Design review of the part built by this model. Coordinates are the model's own, in mm. A direction names the side the tool comes from. Coordinates: 2 decimals unless noted, no trailing zeros. Loops run counter-clockwise (first coordinate to the right, second up) from the corner with the lowest first, then second, coordinate; pieces in that order, holes last. Notation, with made-up numbers: (81.5, 37) - (89.5, 37) arc R16 ccw to (89.5, 55) - close; hole circle Ø8 at (70, 7.5). An arc over 180 degrees is marked (long way). Use one line per item in the form item = value. Start each with the question number.
(1) Add section A-A (z = 14). Count the separate pieces of the cut face and the enclosed holes in it, plus the area to 3 significant figures.
(2) Tool access review of faces 4 (the face through (0.81, 19.37, 26.5)), 5 (the face through (60.85, 1, 14)), 6 (the face through (78.4, 12, 14)): name each direction out of +Z, -Z, +X, -X, +Y, -Y from which nothing blocks a thin tool from reaching the whole face with its end or side.
(3) Add section C-C (x = 39.5). State the section outline as (y, z) points.
(4) The part is to be moulded in two halves that separate along Y. For faces 1 (the face through (39, 1.6, 26)), 2 (the face through (79.189, 14.097, 14.631)), 3 (the face through (0.782, 0.741, 13.804)), say which applies: pulls with the +Y half, pulls with the -Y half, needs draft (parallel to the pull), parting line crosses it, or undercut.
(5) For L1, parallel to Z at x = 78.8, y = 8.1; L2, parallel to X at y = 5, z = 21; L3, parallel to X at y = 1.5, z = 9, list the stretches that pass through material, from the lowest coordinate up.
(6) Clearance check with flat-ended pins moving along their axes: pin 1 Ø4 at (x, z) = (70, 12.5) entering from +Y; pin 2 Ø1.3 at (y, z) = (1, 10) entering from +X; pin 3 Ø5.5 at (x, z) = (65, 18.9) entering from -Y; pin 4 Ø0.8 at (y, z) = (1, 19) entering from +X. State where each tip first meets the part, or that it passes through.
(7) Add section B-B (y = 3.5). State the section outline as (x, z) points, plus the area to 3 significant figures.
(8) Add section D-D (x = 65). State the section outline as (y, z) points, plus the area to 3 significant figures.
```python
from build123d import *

# Parameters (mm, degrees)
SKETCH1_W                      = 80
SKETCH1_H                      = 28
BOSS_EXTRUDE1_DEPTH            = 1.6
SKETCH2_R                      = 2.1
CUT_EXTRUDE1_DEPTH             = 85.77358079
LPATTERN1_COUNT                = 2
LPATTERN1_PITCH                = 50
LPATTERN1_COUNT_DIR2           = 2
LPATTERN1_PITCH_DIR2           = 9.8
SKETCH15_W                     = 41.7
SKETCH15_H                     = 21
CUT_EXTRUDE3_DEPTH             = 85.77358079
EDGE_FLANGE1_STRIP_W           = 8.4
EDGE_FLANGE1_STRIP_H           = 1.6
EDGE_FLANGE1_STRIP_CUT_DEPTH   = 28
EDGE_FLANGE1_STRIP_2_W         = 8.4
EDGE_FLANGE1_STRIP_2_H         = 1.6
EDGE_FLANGE1_STRIP_CUT_2_DEPTH = 28
EDGE_FLANGE1_DEPTH             = 28
EDGE_FLANGE1_BEND_DEPTH        = 28
FILLET1_R                      = 5
SKETCH14_R                     = 2.1
CUT_EXTRUDE2_DEPTH             = 88.273363634
LPATTERN2_COUNT                = 3
LPATTERN2_PITCH                = 8
LPATTERN2_COUNT_DIR2           = 2
LPATTERN2_PITCH_DIR2           = 8
CUT_EXTRUDE4_DEPTH             = 10


# Sheet-metal steps are written as plain solids
with BuildPart() as part:
    # Sketch1 → Boss-Extrude1 (new body)
    with BuildSketch(Plane(origin=(0, 0, 0), x_dir=(1, 0, 0), z_dir=(0, 1, 0))):
        with Locations((40, -14)):
            Rectangle(SKETCH1_W, SKETCH1_H)
    extrude(amount=BOSS_EXTRUDE1_DEPTH)

    # Sketch2 → Cut-Extrude1 (cut, through all)
    with BuildSketch(Plane(origin=(0, 1.6, 0), x_dir=(1, 0, 0), z_dir=(0, 1, 0))):
        with Locations(Location((15, -9.1, 0), (0, 0, 270))):
            Circle(SKETCH2_R)
    cut_extrude1 = extrude(amount=-CUT_EXTRUDE1_DEPTH, mode=Mode.SUBTRACT)

    # LPattern1: Cut-Extrude1 2 × 2
    with Locations(*[(i * LPATTERN1_PITCH, 0, j * LPATTERN1_PITCH_DIR2) for i in range(LPATTERN1_COUNT) for j in range(LPATTERN1_COUNT_DIR2) if (i, j) != (0, 0)]):
        add(cut_extrude1, mode=Mode.SUBTRACT)

    # Sketch15 → Cut-Extrude3 (cut, through all)
    with BuildSketch(Plane(origin=(0, 1.6, 0), x_dir=(1, 0, 0), z_dir=(0, 1, 0))):
        with Locations((40, -14)):
            Rectangle(SKETCH15_W, SKETCH15_H)
    extrude(amount=-CUT_EXTRUDE3_DEPTH, mode=Mode.SUBTRACT)

    # Edge-Flange1 strip (across the edge) → Edge-Flange1 strip cut (cut)
    with BuildSketch(Plane(origin=(80, 1.6, 28), x_dir=(-1, 0, 0), z_dir=(0, 0, -1))):
        with Locations((-1.6, -0.8)):
            Rectangle(EDGE_FLANGE1_STRIP_W, EDGE_FLANGE1_STRIP_H)
    extrude(amount=EDGE_FLANGE1_STRIP_CUT_DEPTH, mode=Mode.SUBTRACT)

    # Edge-Flange1 strip 2 (across the edge) → Edge-Flange1 strip cut 2 (cut)
    with BuildSketch(Plane(origin=(0, 1.6, 0), x_dir=(1, 0, 0), z_dir=(0, 0, 1))):
        with Locations((-1.6, -0.8)):
            Rectangle(EDGE_FLANGE1_STRIP_2_W, EDGE_FLANGE1_STRIP_2_H)
    extrude(amount=EDGE_FLANGE1_STRIP_CUT_2_DEPTH, mode=Mode.SUBTRACT)

    # Edge-Flange1 section (across the edge) → Edge-Flange1 (add)
    with BuildSketch(Plane(origin=(80, 1.6, 28), x_dir=(-1, 0, 0), z_dir=(0, 0, -1))):
        with BuildLine():
            Line((0, 1), (0, 19.2))
            Line((0, 19.2), (1.6, 19.2))
            Line((1.6, 19.2), (1.6, 1))
            ThreePointArc((1.6, 1), (1.892893219, 0.292893219), (2.6, 0))
            Line((2.6, 0), (2.6, -1.6))
            ThreePointArc((2.6, -1.6), (0.761522369, -0.838477631), (0, 1))
        make_face()
    extrude(amount=EDGE_FLANGE1_DEPTH)

    # Edge-Flange1 section 2 (across the edge) → Edge-Flange1 bend (add)
    with BuildSketch(Plane(origin=(0, 1.6, 0), x_dir=(1, 0, 0), z_dir=(0, 0, 1))):
        with BuildLine():
            Line((0, 1), (0, 19.2))
            Line((0, 19.2), (1.6, 19.2))
            Line((1.6, 19.2), (1.6, 1))
            ThreePointArc((1.6, 1), (1.892893219, 0.292893219), (2.6, 0))
            Line((2.6, 0), (2.6, -1.6))
            ThreePointArc((2.6, -1.6), (0.761522369, -0.838477631), (0, 1))
        make_face()
    extrude(amount=EDGE_FLANGE1_BEND_DEPTH)

    # Fillet1
    fillet1_edges = [part.edges().sort_by_distance(p)[0] for p in [
        (79.2, 20.8, 28),
        (79.2, 20.8, 0),
        (0.8, 20.8, 0),
        (0.8, 20.8, 28),
    ]]
    fillet(fillet1_edges, radius=FILLET1_R)

    # Sketch14 → Cut-Extrude2 (cut, through all)
    with BuildSketch(Plane.ZY):
        with Locations(Location((6, 8.1, 0), (0, 0, 270))):
            Circle(SKETCH14_R)
    cut_extrude2 = extrude(amount=-CUT_EXTRUDE2_DEPTH, mode=Mode.SUBTRACT)

    # LPattern2: Cut-Extrude2 3 × 2
    with Locations(*[(0, j * LPATTERN2_PITCH_DIR2, i * LPATTERN2_PITCH) for i in range(LPATTERN2_COUNT) for j in range(LPATTERN2_COUNT_DIR2) if (i, j) != (0, 0)]):
        add(cut_extrude2, mode=Mode.SUBTRACT)

    # Sketch16 → Cut-Extrude4 (cut)
    with BuildSketch(Plane(origin=(0, 1.6, 0), x_dir=(1, 0, 0), z_dir=(0, 1, 0))):
        with BuildLine():
            Line((21.15, -16.1), (17.15, -16.1))
            ThreePointArc((17.15, -16.1), (15.05, -14), (17.15, -11.9))
            Line((17.15, -11.9), (21.15, -11.9))
            ThreePointArc((21.15, -11.9), (23.25, -14), (21.15, -16.1))
        make_face()
    extrude(amount=-CUT_EXTRUDE4_DEPTH, mode=Mode.SUBTRACT)


solid = part.part
```
Computed values:
q1.separate_pieces = 6
q1.enclosed_holes = 0
q1.area = 86.8 mm^2
q2.face_4 = +Z, +X, -X, +Y
q2.face_5 = +Y, -Y
q2.face_6 = +Z, -Z, +Y
q3.outline = (0, 0) - (1.6, 0) - (1.6, 3.5) - (0, 3.5) - close; (0, 24.5) - (1.6, 24.5) - (1.6, 28) - (0, 28) - close
q4.face_1 = pulls with the +Y half
q4.face_2 = undercut
q4.face_3 = pulls with the -Y half
q5.L1 = 0 to 3.9, 8.1 to 11.9, 16.1 to 19.9, 24.1 to 28
q5.L2 = 0 to 1.6, 78.4 to 80
q5.L3 = 0.24 to 12.9, 17.1 to 19.15, 60.85 to 62.9, 67.1 to 79.76
q6.pin_1 = 1.6
q6.pin_2 = 79.82
q6.pin_3 = 0
q6.pin_4 = 79.71
q7.outline = (0, 0) - (1.6, 0) - (1.6, 28) - (0, 28) - close; (78.4, 0) - (80, 0) - (80, 28) - (78.4, 28) - close
q7.area = 89.6 mm^2
q8.outline = (0, 0) - (1.6, 0) - (1.6, 7) - (0, 7) - close; (0, 11.2) - (1.6, 11.2) - (1.6, 16.8) - (0, 16.8) - close; (0, 21) - (1.6, 21) - (1.6, 28) - (0, 28) - close
q8.area = 31.4 mm^2
